Read the model definition and answer for the solid it produces. Units are mm, in the model's axes. Face numbers are marked on the shaded views. A direction names the side the tool comes from. Give positions to 0.01 mm unless a question says otherwise; leave off trailing zeros. Loops run counter-clockwise (first coordinate to the right, second up) from the corner with the lowest first, then second, coordinate; pieces in that order, holes last. Notation, with made-up numbers: (54.5, 67) -> (72.5, 67) arc R17 ccw to (72.5, 84) -> close; hole circle Ø9 at (-12, 5). An arc over 180 degrees is marked (long way). Write each question's results on one line, items separated by ' | '. Start each with the question number.
Item 1: Section A-A on x = 25 is taken. Write down the section's boundary in (y, z).
Item 2: Section C-C on y = 7.5 is taken. Write down the section's boundary in (x, z), and give its area (3 significant figures).
Item 3: Section D-D on z = -25 is taken. Write down the section's boundary in (x, y).
Item 4: Which of the six approach directions +Z, -Z, +X, -X, +Y, -Y give full straight-line access (tool end or side, diameter ignored) to the marked faces 4 and 5?
Item 5: Find the intervals of material crossed by line 1 (X direction, y = 0.8, z = -25); line 2 (X direction, y = 1.4, z = -3); line 3 (X direction, y = 6.75, z = -10.75), in increasing order.
Item 6: Determine the mould class of the marked faces 1, 2 and 3 for opening direction Z: +Z half, -Z half, draft (parallel to the pull), parting line (faces both ways), or undercut.
Item 7: Each of these flat-tipped pins is pushed along its axis until it touches: P1, Ø1.8, axis at x = 3, z = -25, coming from the +Y side; P2, Ø10.5, axis at x = 16, y = 17.5, coming from the -Z side. Where does it stop, or does it pass through?
Item 8: Section B-B on z = -11 is taken. Write down the section's boundary in (x, y).
```python
from build123d import *

# Parameters (mm, degrees)
SKETCH1_W           = 22
SKETCH1_H           = 22
SKETCH1_R           = 7.5
BOSS_EXTRUDE1_DEPTH = 24
SKETCH2_R           = 1.5
BOSS_EXTRUDE2_DEPTH = 3


with BuildPart() as part:
    # Sketch1 → Boss-Extrude1 (new body)
    with BuildSketch(Plane(origin=(0, 0, 0), x_dir=(1, 0, 0), z_dir=(0, 1, 0))):
        with Locations((11, 11)):
            Rectangle(SKETCH1_W, SKETCH1_H)
        with Locations(Location((11, 11, 0), (0, 0, 270))):
            Circle(SKETCH1_R, mode=Mode.SUBTRACT)
    extrude(amount=BOSS_EXTRUDE1_DEPTH)

    # Sketch2 → Boss-Extrude2 (add)
    with BuildSketch(Plane.XZ):
        Polygon((0, -22), (22, -22), (22, 0), (28, 0), (28, -28), (0, -28), align=None)
        with Locations(Location((25, -25, 0), (0, 0, 270))):
            Circle(SKETCH2_R, mode=Mode.SUBTRACT)
        with Locations(Location((25, -3, 0), (0, 0, 270))):
            Circle(SKETCH2_R, mode=Mode.SUBTRACT)
        with Locations(Location((3, -25, 0), (0, 0, 270))):
            Circle(SKETCH2_R, mode=Mode.SUBTRACT)
    extrude(amount=-BOSS_EXTRUDE2_DEPTH)


solid = part.part
```
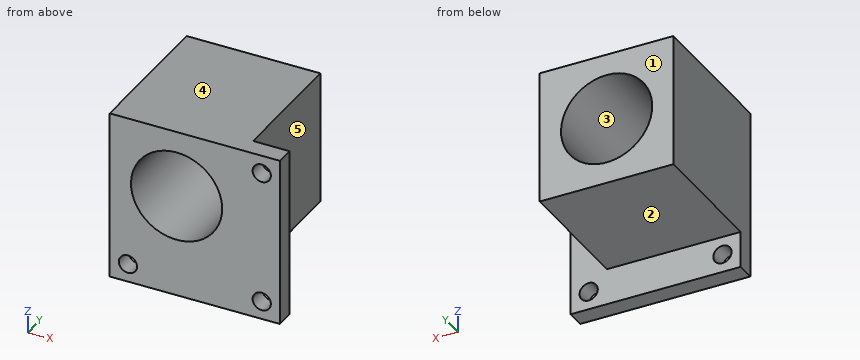
Findings:
1) outline: (0, -28) -> (3, -28) -> (3, -26.5) -> (0, -26.5) -> close; (0, -23.5) -> (3, -23.5) -> (3, -4.5) -> (0, -4.5) -> close; (0, -1.5) -> (3, -1.5) -> (3, 0) -> (0, 0) -> close
2) outline: (0, -22) -> (22, -22) -> (22, 0) -> (0, 0) -> close; hole circle Ø15 at (11, -11) | area: 307 mm2
3) outline: (0, 0) -> (1.5, 0) -> (1.5, 3) -> (0, 3) -> close; (4.5, 0) -> (23.5, 0) -> (23.5, 3) -> (4.5, 3) -> close; (26.5, 0) -> (28, 0) -> (28, 3) -> (26.5, 3) -> close
4) face 4: +Z, +X, -X, +Y, -Y | face 5: +Z, -Z, +X, +Y
5) line 1: 0 to 1.5, 4.5 to 23.5, 26.5 to 28 | line 2: 0 to 23.5, 26.5 to 28 | line 3: 0 to 3.5, 18.5 to 22
6) face 1: draft | face 2: -Z half | face 3: undercut
7) P1: through | P2: z = -22
8) outline: (0, 0) -> (3.5, 0) -> (3.5, 24) -> (0, 24) -> close; (18.5, 0) -> (28, 0) -> (28, 3) -> (22, 3) -> (22, 24) -> (18.5, 24) -> close
